from build123d import *

# Parameters (mm, degrees)
F0_R     = 76.2
F1_DEPTH = 19.05
F2_R     = 57.205145
F3_DEPTH = 12.7
F4_R     = 5.08
F5_R     = 5.08


with BuildPart() as f1:
    # F0 (on Top) → F1 (new body)
    with BuildSketch(Plane.XY):
        Circle(F0_R)
    extrude(amount=F1_DEPTH)

    # F2 (on face) → F3 (cut)
    with BuildSketch(Plane.XY.offset(19.05)):
        Circle(F2_R)
    extrude(amount=-F3_DEPTH, mode=Mode.SUBTRACT)

    # F4
    f4_edges = [f1.edges().sort_by_distance(p)[0] for p in [
        (-57.205145, 0, 19.05),
        (-76.2, 0, 19.05),
    ]]
    fillet(f4_edges, radius=F4_R)

    # F5
    f5_edges = [f1.edges().sort_by_distance(p)[0] for p in [
        (-76.2, 0, 0),
    ]]
    fillet(f5_edges, radius=F5_R)


solid = f1.part
The model under review builds one solid part; all positions refer to its coordinate system, in mm. A direction names the side the tool comes from. Coordinates: 2 decimals unless noted, no trailing zeros. Write each loop counter-clockwise with the first axis right and the second up, starting at its lowest first coordinate (ties: lowest second). Pieces come first, ordered by that corner, then holes. Notation, with made-up numbers: (34.5, 88) - (64.5, 88) arc R29 ccw to (64.5, 111) - close; hole circle Ø8 at (9.25, -35.75). An arc over 180 degrees is marked (long way). Answer as CSV lines item,"result".
(1) Clearance check with flat-ended pins moving along their axes: pin 1 Ø5 at (x, z) = (37.5, 16) entering from -Y; pin 2 Ø10 at (x, z) = (1, 4.5) entering from +Y; pin 3 Ø4 at (y, z) = (56.5, 13.5) entering from +X. State where each tip first meets the part, or that it passes through.
Data:
pin 1,"stops at y = -67.46"
pin 2,"stops at y = 76.2"
pin 3,"stops at x = 53.26"
(2) Mouldability with a two-part tool opening along Y and no side actions: class faces 3 (the cylindrical face through (26.4, -50.75, 10.21)), 4 (the cylindrical face through (-60.47, -46.367, 9.463)), 5 (the flat face through (-1, 1, 0)) as pulls with the +Y half, pulls with the -Y half, needs draft (parallel to the pull), parting line crosses it, or undercut.
Data:
face 3,"undercut"
face 4,"parting line crosses it"
face 5,"needs draft"
(3) Tool access review of faces 1 (the flat face through (0, -63, 19.05)), 2 (the flat face through (-1, 1, 6.35)): name each direction out of +Z, -Z, +X, -X, +Y, -Y from which nothing blocks a thin tool from reaching the whole face with its end or side.
Data:
face 1,"+Z, +X, -X, +Y, -Y"
face 2,"+Z"
(4) We need section C-C (z = 9). Give the boundary of the cut face in (x, y), plus the area to 3 significant figures.
Data:
outline,"circle Ø152.4 at (0, 0); hole circle Ø114.41 at (0, 0)"
area,"7,960 mm2"
(5) For line 1 along Y through (x, z) = (0, 12.5); line 2 along X through (y, z) = (18.5, 10.25); line 3 along Z through (x, y) = (-41.5, 24), list the stretches that pass through material, from the lowest coordinate up. Write a range as [from, to].
Data:
line 1,"y = [-76.2, -57.21], [57.21, 76.2]"
line 2,"x = [-73.92, -54.13], [54.13, 73.92]"
line 3,"z = [0, 6.35]"
(6) We need section A-A (x = 0). Give the boundary of the cut face in (y, z), plus the area to 3 significant figures.
Data:
outline,"(-76.2, 5.08) arc R5.08 ccw to (-71.12, 0) - (71.12, 0) arc R5.08 ccw to (76.2, 5.08) - (76.2, 13.97) arc R5.08 ccw to (71.12, 19.05) - (62.29, 19.05) arc R5.08 ccw to (57.21, 13.97) - (57.21, 6.35) - (-57.21, 6.35) - (-57.21, 13.97) arc R5.08 ccw to (-62.29, 19.05) - (-71.12, 19.05) arc R5.08 ccw to (-76.2, 13.97) - close"
area,"1,420 mm2"
